Could you check a few things on this model? Use its own coordinates, in mm. Face numbers are marked on the shaded views. A direction names the side the tool comes from. Round coordinates to 2 decimals unless told otherwise and drop trailing zeros. Order: outer loops, then holes, each group sorted by start corner. A loop starts at its lowest first (then second) coordinate and runs counter-clockwise, first axis right, second up. Notation, with made-up numbers: (-11.5, -20) -> (32.5, -20) arc R27 ccw to (32.5, 10) -> close; hole circle Ø7 at (36.5, -13). An arc over 180 degrees is marked (long way). One line per question, with ' | ' between items.
```python
from build123d import *

# Parameters (mm, degrees)
BOSS_EXTRUDE1_DEPTH    = 58
SKETCH25_R             = 4
CUT_EXTRUDE6_DEPTH     = 10
SKETCH26_W             = 103.5
SKETCH26_H             = 2
CUT_EXTRUDE7_DEPTH     = 90
SKETCH29_R             = 1.5
CUT_EXTRUDE8_DEPTH     = 10
CONVERT_SOLID1_DEPTH   = 58
CONVERT_SOLID1_2_DEPTH = 58
SKETCH2_R              = 2.5
SKETCH2_R_2            = 20
CUT_EXTRUDE10_DEPTH    = 10
SKETCH30_R             = 3.5
CUT_EXTRUDE11_DEPTH    = 10


# Read off the part's stored shape, not the designer's step: Convert-Solid1
with BuildPart() as part:
    # Sketch1 → Boss-Extrude1 (new body)
    with BuildSketch(Plane(origin=(0, 0, 0), x_dir=(0, 0, -1), z_dir=(1, 0, 0))):
        Polygon((-73.351671883, 30.400809615), (-73.351671883, -29.599190385), (30.148328117, -29.599190385), (30.148328117, 30.400809615), (33.148328117, 30.400809615), (33.148328117, -34.599190385), (-76.351671883, -34.599190385), (-76.351671883, 30.400809615), align=None)
    extrude(amount=BOSS_EXTRUDE1_DEPTH)

    # Sketch25 → Cut-Extrude6 (cut)
    with BuildSketch(Plane.XZ.offset(34.599190385)):
        with Locations(Location((29, 20.601671883, 0), (0, 0, 270))):
            Circle(SKETCH25_R)
    extrude(amount=-CUT_EXTRUDE6_DEPTH, mode=Mode.SUBTRACT)

    # Sketch26 → Cut-Extrude7 (cut)
    with BuildSketch(Plane(origin=(58, 0, 0), x_dir=(0, 0, -1), z_dir=(1, 0, 0))):
        with Locations((-21.601671883, -30.599190385)):
            Rectangle(SKETCH26_W, SKETCH26_H)
    extrude(amount=-CUT_EXTRUDE7_DEPTH, mode=Mode.SUBTRACT)

    # Sketch29 → Cut-Extrude8 (cut)
    with BuildSketch(Plane(origin=(0, -31.599190385, 0), x_dir=(1, 0, 0), z_dir=(0, 1, 0))):
        with Locations(Location((19.5, -20.601671883, 0), (0, 0, 270))):
            Circle(SKETCH29_R)
        with Locations(Location((24.25, -12.374430547, 0), (0, 0, 270))):
            Circle(SKETCH29_R)
        with Locations(Location((33.75, -12.374430547, 0), (0, 0, 270))):
            Circle(SKETCH29_R)
        with Locations(Location((38.5, -20.601671883, 0), (0, 0, 270))):
            Circle(SKETCH29_R)
        with Locations(Location((33.75, -28.828913219, 0), (0, 0, 270))):
            Circle(SKETCH29_R)
        with Locations(Location((24.25, -28.828913219, 0), (0, 0, 270))):
            Circle(SKETCH29_R)
    extrude(amount=-CUT_EXTRUDE8_DEPTH, mode=Mode.SUBTRACT)

    # Convert-Solid1 outline → Convert-Solid1 (cut)
    with BuildSketch(Plane.YZ):
        with BuildLine():
            Line((-34.599190385, -33.148328117), (-29.599190385, -33.148328117))
            ThreePointArc((-29.599190385, -33.148328117), (-33.134724291, -31.683862023), (-34.599190385, -28.148328117))
            Line((-34.599190385, -28.148328117), (-34.599190385, -33.148328117))
        make_face()
        with BuildLine():
            Line((-34.599190385, 76.351671883), (-34.599190385, 71.351671883))
            ThreePointArc((-34.599190385, 71.351671883), (-33.134724291, 74.887205789), (-29.599190385, 76.351671883))
            Line((-29.599190385, 76.351671883), (-34.599190385, 76.351671883))
        make_face()
    extrude(amount=CONVERT_SOLID1_DEPTH, mode=Mode.SUBTRACT)

    # Convert-Solid1 2 outline → Convert-Solid1 2 (add)
    with BuildSketch(Plane.YZ):
        with BuildLine():
            Line((-31.599190385, -30.148328117), (-29.599190385, -30.148328117))
            ThreePointArc((-29.599190385, -30.148328117), (-31.013403947, -29.56254168), (-31.599190385, -28.148328117))
            Line((-31.599190385, -28.148328117), (-31.599190385, -30.148328117))
        make_face()
        with BuildLine():
            Line((-31.599190385, 73.351671883), (-31.599190385, 71.351671883))
            ThreePointArc((-31.599190385, 71.351671883), (-31.013403947, 72.765885445), (-29.599190385, 73.351671883))
            Line((-29.599190385, 73.351671883), (-31.599190385, 73.351671883))
        make_face()
    extrude(amount=CONVERT_SOLID1_2_DEPTH)

    # Sketch2 → Cut-Extrude10 (cut)
    with BuildSketch(Plane.XY.offset(76.351671883)):
        with Locations((5.5, 24.900809615)):
            Circle(SKETCH2_R)
        with Locations(Location((52.5, 24.900809615, 0), (0, 0, 270))):
            Circle(SKETCH2_R)
        with Locations((52.5, -22.099190385)):
            Circle(SKETCH2_R)
        with Locations(Location((5.5, -22.099190385, 0), (0, 0, 270))):
            Circle(SKETCH2_R)
        with Locations((29, 1.400809615)):
            Circle(SKETCH2_R_2)
    extrude(amount=-CUT_EXTRUDE10_DEPTH, mode=Mode.SUBTRACT)

    # Sketch30 → Cut-Extrude11 (cut)
    with BuildSketch(Plane(origin=(0, 0, -33.148328117), x_dir=(-1, 0, 0), z_dir=(0, 0, -1))):
        with Locations((-29, 1.400809615)):
            Circle(SKETCH30_R)
    extrude(amount=-CUT_EXTRUDE11_DEPTH, mode=Mode.SUBTRACT)


solid = part.part
```
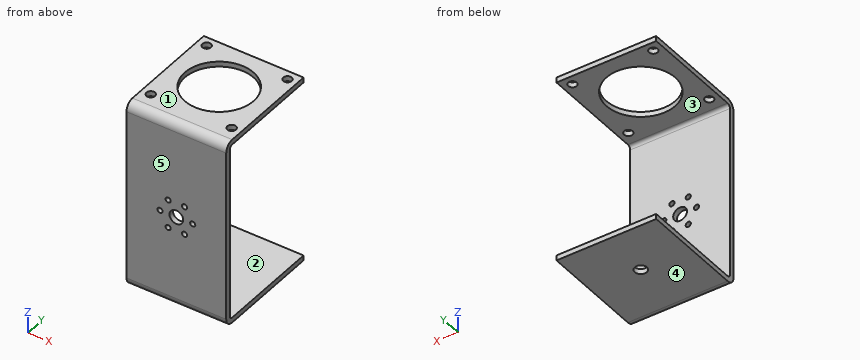
1. I want a section at B-B on x = 5.5. List the corners of the cut face in (y, z) for me.
From the geometry:
outline: (-34.6, -28.15) arc R5 ccw to (-29.6, -33.15) -> (30.4, -33.15) -> (30.4, -30.15) -> (-29.6, -30.15) arc R2 cw to (-31.6, -28.15) -> (-31.6, 71.35) arc R2 cw to (-29.6, 73.35) -> (-24.6, 73.35) -> (-24.6, 76.35) -> (-29.6, 76.35) arc R5 ccw to (-34.6, 71.35) -> close; (-19.6, 73.35) -> (22.4, 73.35) -> (22.4, 76.35) -> (-19.6, 76.35) -> close; (27.4, 73.35) -> (30.4, 73.35) -> (30.4, 76.35) -> (27.4, 76.35) -> close
2. I need wall thicknesses on probe 1 along Z at (x, y) = (54.5, 7); probe 2 along Y at (x, z) = (5.5, 0); probe 3 along Z at (x, y) = (19, -7). Which ranges of each line are inside material? Lowest first, please.
From the geometry:
probe 1: z = -33.15 to -30.15, 73.35 to 76.35 | probe 2: y = -34.6 to -31.6 | probe 3: z = -33.15 to -30.15
3. On a 3-axis mill with a long thin cutter (end or side, diameter ignored), from which of +Z, -Z, +X, -X, +Y, -Y can I reach the whole of each face in a straight line? I mean the marked faces 1 and 2. Say none if no direction works.
From the geometry:
face 1: +Z, +X, -X, +Y, -Y | face 2: +X, -X, +Y
4. I want a section at A-A on x = 29. List the corners of the cut face in (y, z) for me.
From the geometry:
outline: (-34.6, -28.15) arc R5 ccw to (-29.6, -33.15) -> (-2.1, -33.15) -> (-2.1, -30.15) -> (-29.6, -30.15) arc R2 cw to (-31.6, -28.15) -> (-31.6, 16.6) -> (-34.6, 16.6) -> close; (-34.6, 24.6) -> (-31.6, 24.6) -> (-31.6, 71.35) arc R2 cw to (-29.6, 73.35) -> (-18.6, 73.35) -> (-18.6, 76.35) -> (-29.6, 76.35) arc R5 ccw to (-34.6, 71.35) -> close; (4.9, -33.15) -> (30.4, -33.15) -> (30.4, -30.15) -> (4.9, -30.15) -> close; (21.4, 73.35) -> (30.4, 73.35) -> (30.4, 76.35) -> (21.4, 76.35) -> close
5. I'm going to push flat-ended pins straight in: pin 1 (5 mm diameter, centred on x = 24.25, z = 28.83, fed in from +Y); pin 2 (4.5 mm diameter, centred on x = 5.5, y = -22.1, fed in from +Z); pin 3 (6.5 mm diameter, centred on x = 29, z = 20.6, fed in from -Y). Where does each tip first touch, or does it pass through?
From the geometry:
pin 1: stops at y = -31.6 | pin 2: stops at z = -30.15 | pin 3: passes through
6. I want a section at C-C on y = -27. List the corners of the cut face in (x, z) for me.
From the geometry:
outline: (0, -33.15) -> (58, -33.15) -> (58, -30.15) -> (0, -30.15) -> close; (0, 73.35) -> (58, 73.35) -> (58, 76.35) -> (0, 76.35) -> close
7. I want a section at D-D on x = 45.5. List the corners of the cut face in (y, z) for me.
From the geometry:
outline: (-34.6, -28.15) arc R5 ccw to (-29.6, -33.15) -> (30.4, -33.15) -> (30.4, -30.15) -> (-29.6, -30.15) arc R2 cw to (-31.6, -28.15) -> (-31.6, 71.35) arc R2 cw to (-29.6, 73.35) -> (-9.9, 73.35) -> (-9.9, 76.35) -> (-29.6, 76.35) arc R5 ccw to (-34.6, 71.35) -> close; (12.7, 73.35) -> (30.4, 73.35) -> (30.4, 76.35) -> (12.7, 76.35) -> close
8. If we mould it in two halves opening along Z, with no side actions, what happens to the marked faces 3, 4 and 5? For each: pulls with the +Z half, pulls with the -Z half, needs draft (parallel to the pull), parting line crosses it, or undercut.
From the geometry:
face 3: undercut | face 4: pulls with the -Z half | face 5: needs draft
